The model under review builds one solid part; all positions refer to its coordinate system, in mm. A direction names the side the tool comes from. Give positions to 0.01 mm unless a question says otherwise; leave off trailing zeros. Loops run counter-clockwise (first coordinate to the right, second up) from the corner with the lowest first, then second, coordinate; pieces in that order, holes last. Notation, with made-up numbers: M -4,17.5 L 32,17.5 A16 ccw 32,40.5 Z; hole C 35.25,33 d2. An arc over 180 degrees is marked long. Return JSON: item names as keys, results as strings. Group by question number.
```python
from build123d import *

# Parameters (mm, degrees)
SKETCH1_W           = 210
SKETCH1_H           = 50
SKETCH1_R           = 1.211665018
SKETCH1_R_2         = 1.165617118
SKETCH1_R_3         = 1.5
SKETCH1_R_4         = 1.25
SKETCH1_R_5         = 1.517273905
SKETCH1_R_6         = 3.4
BOSS_EXTRUDE1_DEPTH = 3.175
SKETCH2_R           = 2
CUT_EXTRUDE1_DEPTH  = 10
SKETCH3_R           = 6
SKETCH3_R_2         = 0.586995366
CUT_EXTRUDE2_DEPTH  = 57.15
CUT_EXTRUDE7_DEPTH  = 10
FILLET3_R           = 5
SKETCH11_R          = 18.5
SKETCH11_R_2        = 2
BOSS_EXTRUDE4_DEPTH = 3.175
SKETCH16_W          = 18.257640281
SKETCH16_H          = 3.175
BOSS_EXTRUDE7_DEPTH = 8.128
SKETCH17_W          = 33.3
SKETCH17_H          = 3.175
BOSS_EXTRUDE8_DEPTH = 35.56
SKETCH18_R          = 2
CUT_EXTRUDE8_DEPTH  = 9
SKETCH19_R          = 4
CUT_EXTRUDE9_DEPTH  = 40
FILLET4_R           = 5
SKETCH20_R          = 3.5
CUT_EXTRUDE10_DEPTH = 10
SKETCH21_R          = 1.5
CUT_EXTRUDE11_DEPTH = 10
SKETCH22_R          = 1.5
CUT_EXTRUDE12_DEPTH = 10
SKETCH24_R          = 1.5
CUT_EXTRUDE13_DEPTH = 10


with BuildPart() as part:
    # Sketch1 → Boss-Extrude1 (new body)
    with BuildSketch(Plane(origin=(0, 0, 0), x_dir=(1, 0, 0), z_dir=(0, 1, 0))):
        with Locations((105, -25)):
            Rectangle(SKETCH1_W, SKETCH1_H)
        with Locations(Location((3.489526233, -16.787661112, 0), (0, 0, 270))):
            Circle(SKETCH1_R, mode=Mode.SUBTRACT)
        with Locations(Location((34.37258772, -17.194005245, 0), (0, 0, 270))):
            Circle(SKETCH1_R_2, mode=Mode.SUBTRACT)
        with Locations(Location((37.520749958, -44.921198121, 0), (0, 0, 270))):
            Circle(SKETCH1_R_3, mode=Mode.SUBTRACT)
        with Locations(Location((122, -42.058139805, 0), (0, 0, 270))):
            Circle(SKETCH1_R_4, mode=Mode.SUBTRACT)
        with Locations(Location((168.975233936, -37.403209633, 0), (0, 0, 270))):
            Circle(SKETCH1_R_5, mode=Mode.SUBTRACT)
        with Locations(Location((18, -34, 0), (0, 0, 270))):
            Circle(SKETCH1_R_6, mode=Mode.SUBTRACT)
    extrude(amount=BOSS_EXTRUDE1_DEPTH)

    # Sketch2 → Cut-Extrude1 (cut)
    with BuildSketch(Plane(origin=(0, 3.175, 0), x_dir=(1, 0, 0), z_dir=(0, 1, 0))):
        with Locations(Location((10, -26, 0), (0, 0, 270))):
            Circle(SKETCH2_R)
        with Locations(Location((10, -42, 0), (0, 0, 270))):
            Circle(SKETCH2_R)
        with Locations(Location((26, -26, 0), (0, 0, 270))):
            Circle(SKETCH2_R)
        with Locations(Location((26, -42, 0), (0, 0, 270))):
            Circle(SKETCH2_R)
    extrude(amount=-CUT_EXTRUDE1_DEPTH, mode=Mode.SUBTRACT)

    # Sketch3 → Cut-Extrude2 (cut)
    with BuildSketch(Plane(origin=(0, 3.175, 0), x_dir=(1, 0, 0), z_dir=(0, 1, 0))):
        with Locations(Location((78.01026379, -28.1, 0), (0, 0, 270))):
            Circle(SKETCH3_R)
        with Locations(Location((145.531297368, -14, 0), (0, 0, 270))):
            Circle(SKETCH3_R)
        with Locations((18, -34)):
            Circle(SKETCH3_R_2)
        with Locations(Location((202.646291021, -16, 0), (0, 0, 270))):
            Circle(SKETCH3_R)
    extrude(amount=-CUT_EXTRUDE2_DEPTH, mode=Mode.SUBTRACT)

    # Sketch10 → Cut-Extrude7 (cut)
    with BuildSketch(Plane(origin=(0, 3.175, 0), x_dir=(1, 0, 0), z_dir=(0, 1, 0))):
        Polygon((210, -27.859435908), (165.502877994, -50), (210, -50), align=None)
        Polygon((92.532613397, 0), (77.65477062, -7.402812063), (0, -7.402812063), (0, 0), align=None)
    extrude(amount=-CUT_EXTRUDE7_DEPTH, mode=Mode.SUBTRACT)

    # Fillet3
    fillet3_edges = [part.edges().sort_by_distance(p)[0] for p in [
        (210, 1.5875, 0),
        (92.532613397, 1.5875, 0),
        (210, 1.5875, 27.859435908),
        (165.502877994, 1.5875, 50),
        (77.65477062, 1.5875, 7.402812063),
    ]]
    fillet(fillet3_edges, radius=FILLET3_R)

    # Sketch11 → Boss-Extrude4 (add)
    with BuildSketch(Plane(origin=(0, 3.175, 0), x_dir=(1, 0, 0), z_dir=(0, 1, 0))):
        with Locations((18, -34)):
            Circle(SKETCH11_R)
        with Locations(Location((10, -26, 0), (0, 0, 270))):
            Circle(SKETCH11_R_2, mode=Mode.SUBTRACT)
        with Locations(Location((10, -42, 0), (0, 0, 270))):
            Circle(SKETCH11_R_2, mode=Mode.SUBTRACT)
        with Locations(Location((26, -26, 0), (0, 0, 270))):
            Circle(SKETCH11_R_2, mode=Mode.SUBTRACT)
        with Locations(Location((26, -42, 0), (0, 0, 270))):
            Circle(SKETCH11_R_2, mode=Mode.SUBTRACT)
    extrude(amount=-BOSS_EXTRUDE4_DEPTH)

    # Sketch16 → Boss-Extrude7 (add)
    with BuildSketch(Plane(origin=(0, 0, 7.402812063), x_dir=(-1, 0, 0), z_dir=(0, 0, -1))):
        with Locations((-9.128820141, 1.5875)):
            Rectangle(SKETCH16_W, SKETCH16_H)
    extrude(amount=BOSS_EXTRUDE7_DEPTH)

    # Sketch17 → Boss-Extrude8 (add)
    with BuildSketch(Plane.ZY):
        with Locations((15.924812063, 1.5875)):
            Rectangle(SKETCH17_W, SKETCH17_H)
    extrude(amount=BOSS_EXTRUDE8_DEPTH)

    # Sketch18 → Cut-Extrude8 (cut)
    with BuildSketch(Plane(origin=(0, 3.175, 0), x_dir=(1, 0, 0), z_dir=(0, 1, 0))):
        with Locations(Location((-29.612034681, -23.798543698, 0), (0, 0, 270))):
            Circle(SKETCH18_R)
        with Locations(Location((-29.359661767, -7.798707515, 0), (0, 0, 270))):
            Circle(SKETCH18_R)
        with Locations(Location((-13.359825583, -8.051080428, 0), (0, 0, 270))):
            Circle(SKETCH18_R)
        with Locations(Location((-13.612198497, -24.050916612, 0), (0, 0, 270))):
            Circle(SKETCH18_R)
    extrude(amount=-CUT_EXTRUDE8_DEPTH, mode=Mode.SUBTRACT)

    # Sketch19 → Cut-Extrude9 (cut)
    with BuildSketch(Plane(origin=(0, 3.175, 0), x_dir=(1, 0, 0), z_dir=(0, 1, 0))):
        with Locations(Location((-21.359661767, -15.798707515, 0), (0, 0, 270))):
            Circle(SKETCH19_R)
    extrude(amount=-CUT_EXTRUDE9_DEPTH, mode=Mode.SUBTRACT)

    # Fillet4
    fillet4_edges = [part.edges().sort_by_distance(p)[0] for p in [
        (18.257640281, 1.5875, -0.725187937),
        (-35.56, 1.5875, -0.725187937),
        (-35.56, 1.5875, 32.574812063),
        (0, 1.5875, 50),
    ]]
    fillet(fillet4_edges, radius=FILLET4_R)

    # Sketch20 → Cut-Extrude10 (cut)
    with BuildSketch(Plane(origin=(0, 3.175, 0), x_dir=(1, 0, 0), z_dir=(0, 1, 0))):
        with Locations(Location((18, -34, 0), (0, 0, 270))):
            Circle(SKETCH20_R)
    extrude(amount=-CUT_EXTRUDE10_DEPTH, mode=Mode.SUBTRACT)

    # Sketch21 → Cut-Extrude11 (cut)
    with BuildSketch(Plane(origin=(0, 3.175, 0), x_dir=(1, 0, 0), z_dir=(0, 1, 0))):
        with Locations(Location((116, -4.237214774, 0), (0, 0, 270))):
            Circle(SKETCH21_R)
    extrude(amount=-CUT_EXTRUDE11_DEPTH, mode=Mode.SUBTRACT)

    # Sketch22 → Cut-Extrude12 (cut)
    with BuildSketch(Plane(origin=(0, 3.175, 0), x_dir=(1, 0, 0), z_dir=(0, 1, 0))):
        with Locations(Location((12.257640281, -3.274812063, 0), (0, 0, 270))):
            Circle(SKETCH22_R)
    extrude(amount=-CUT_EXTRUDE12_DEPTH, mode=Mode.SUBTRACT)

    # Sketch24 → Cut-Extrude13 (cut)
    with BuildSketch(Plane(origin=(0, 3.175, 0), x_dir=(1, 0, 0), z_dir=(0, 1, 0))):
        with Locations(Location((-30.56, -15.774812063, 0), (0, 0, 270))):
            Circle(SKETCH24_R)
    extrude(amount=-CUT_EXTRUDE13_DEPTH, mode=Mode.SUBTRACT)


solid = part.part
```
(1) For pin 1 (3 mm diameter, centred on x = 26, z = 26, fed in from -Y); pin 2 (1.5 mm diameter, centred on x = 130.5, y = 2, fed in from +Z), all flat-tipped, find the tip position at first contact; note any pin that passes through.
(2) Mouldability with a two-part tool opening along X and no side actions: class faces 1 (the cylindrical face through (208, 2, 1)), 2 (the flat face through (89, 0, 26)), 3 (the cylindrical face through (-13.01, 1.61, 25.96)) as released by +X, released by -X, zero draft, split by the parting line, or undercut.
(3) For probe 1 along X at (y, z) = (1.55, 36.5); probe 2 along X at (y, z) = (2.7, 3); probe 3 along X at (y, z) = (1.6, 2.5), list the stretches that pass through material, from the lowest coordinate up.
(4) Add section C-C (x = 182.5). Write out the cut boundary in (y, z) (3 decimals).
(5) For faces 4 (the flat face through (187.176, 1.61, 39.216)), 5 (the flat face through (85.18, 1.61, 3.66)), list the 3-axis set-ups (+Z, -Z, +X, -X, +Y, -Y) from which the entire face can be reached by the end or side of a thin tool; tool diameter is ignored.
(6) Add section B-B (y = 2.15). Count the separate pieces of the cut face and the enclosed holes in it, and give its area (3 significant figures).
(7) Add section A-A (x = -5.5). Write out the cut boundary in (y, z) (3 decimals).
Verdict:
{
 "1": {"pin 1": "passes through", "pin 2": "stops at z = 50"},
 "2": {"face 1": "released by +X", "face 2": "zero draft", "face 3": "undercut"},
 "3": {"probe 1": "x = -0.33 to 15.55, 20.45 to 167.76, 170.19 to 192.63", "probe 2": "x = -35.39 to 10.78, 13.73 to 18.09, 86.5 to 115.15, 116.85 to 209.58", "probe 3": "x = -35.23 to 10.97, 13.54 to 17.93, 87.51 to 209.33"},
 "4": {"outline": "M 0,0 L 3.175,0 L 3.175,41.543 L 0,41.543 Z"},
 "5": {"face 4": "+Z, +X, +Y, -Y", "face 5": "-Z, +Y, -Y"},
 "6": {"separate pieces": "1", "enclosed holes": "21", "area": "10,100 mm²"},
 "7": {"outline": "M 0,-0.725 L 3.175,-0.725 L 3.175,32.575 L 0,32.575 Z"}
}
